```python
from build123d import *

# Parameters (mm, degrees)
SKETCH4_R                = 150
BOSS_EXTRUDE1_DEPTH      = 25
BOSS_EXTRUDE1_DEPTH_BACK = 25
SKETCH4_4_R              = 230
SKETCH4_4_R_2            = 150
BOSS_EXTRUDE2_DEPTH      = 25


with BuildPart() as part:
    # Sketch4 → Boss-Extrude1 (new body, two sides)
    with BuildSketch(Plane.XY) as boss_extrude1_sk:
        with BuildLine():
            Line((71.8245835, 175.909198012), (-101.8245835, 175.909198012))
            ThreePointArc((-101.8245835, 175.909198012), (-480, 0), (-101.8245835, -175.909198012))
            Line((-101.8245835, -175.909198012), (71.8245835, -175.909198012))
            ThreePointArc((71.8245835, -175.909198012), (450, 0), (71.8245835, 175.909198012))
        make_face()
        with Locations((-250, 0)):
            Circle(SKETCH4_R, mode=Mode.SUBTRACT)
        with Locations((220, 0)):
            Circle(SKETCH4_R, mode=Mode.SUBTRACT)
    extrude(amount=BOSS_EXTRUDE1_DEPTH)
    extrude(boss_extrude1_sk.sketch, amount=-BOSS_EXTRUDE1_DEPTH_BACK)

    # Sketch4_4 → Boss-Extrude2 (add)
    with BuildSketch(Plane.XY):
        with Locations((-250, 0)):
            Circle(SKETCH4_4_R)
        with Locations((-250, 0)):
            Circle(SKETCH4_4_R_2, mode=Mode.SUBTRACT)
        with Locations((220, 0)):
            Circle(SKETCH4_4_R)
        with Locations((220, 0)):
            Circle(SKETCH4_4_R_2, mode=Mode.SUBTRACT)
    extrude(amount=-BOSS_EXTRUDE2_DEPTH)


solid = part.part
```
Geometry: final body of the model. Coordinates: model frame, mm. A direction names the side the tool comes from. Coordinates: 2 decimals unless noted, no trailing zeros. Write each loop counter-clockwise with the first axis right and the second up, starting at its lowest first coordinate (ties: lowest second). Pieces come first, ordered by that corner, then holes. Notation, with made-up numbers: M 6.25,82 L 27.25,82 A16 cw 27.25,109 Z; hole C 6.25,36.5 d3. An arc over 180 degrees is marked long. Answer as CSV lines item,"result". Start each with the question number.
Q1. Cut plane B-B on y = -71. Return the cut outline in (x, z), then the cut area to 3 significant figures.
Q2. Reachability of faces 4 (the flat face through (-16, -175.909, 0)), 5 (the flat face through (-14, 175.909, 0)), 6 (the cylindrical face through (-106.93, 45.06, -0.35)) from +Z, -Z, +X, -X, +Y, -Y: full face, straight path, thin tool, end or side. Return the list, or none.
Q3. Mould query, pull axis Y, two halves, no side actions, for faces 1 (the flat face through (-22, 3, 25)), 2 (the cylindrical face through (-479.884, 7.311, 0.35)), 3 (the cylindrical face through (363.07, 45.06, -0.35)). Classes: released by +Y, released by -Y, zero draft, split by the parting line, or undercut.
Q4. Cut plane C-C on z = 16. Return the cut outline in (x, y), then the cut area to 3 significant figures.
Q5. Line query: line 1 (X direction, y = -1, z = 18.5); line 2 (Y direction, x = 220, z = 13.5); line 3 (X direction, y = -12.5, z = 1.5). Output: solid intervals per line, ascending. Write a range as from..to.
Q6. Cut plane A-A on x = 220. Return the cut outline in (y, z), then the cut area to 3 significant figures.
Q7. Cut plane D-D on y = 191.5. Return the cut outline in (x, z).
Q8. Pin query (flat end, axial travel): P1, Ø15, axis at x = 28.5, z = -6, coming from the -Y side; P2, Ø1.5, axis at x = 116, z = 9.5, coming from the -Y side; P3, Ø10, axis at y = -161, z = -12, coming from the +X side. Return the tip coordinate at first contact, or that it passes through.
Findings below:
1,outline,"M -468.77,-25 L -382.13,-25 L -382.13,25 L -468.77,25 Z; M -117.87,-25 L 87.87,-25 L 87.87,25 L -117.87,25 Z; M 352.13,-25 L 438.77,-25 L 438.77,25 L 352.13,25 Z"
1,area,"19,000 mm2"
2,face 4,"+Z, -Z, -Y"
2,face 5,"+Z, -Z, +Y"
2,face 6,"+Z, -Z"
3,face 1,"zero draft"
3,face 2,"split by the parting line"
3,face 3,"undercut"
4,outline,"M -101.82,-175.91 L 71.82,-175.91 A230 ccw long 71.82,175.91 L -101.82,175.91 A230 ccw long Z; hole C -250,0 d300; hole C 220,0 d300"
4,area,"212,000 mm2"
5,line 1,"x = -480..-400, -100..70, 370..450"
5,line 2,"y = -230..-150, 150..230"
5,line 3,"x = -479.66..-399.48, -100.52..70.52, 369.48..449.66"
6,outline,"M -230,-25 L -150,-25 L -150,25 L -230,25 Z; M 150,-25 L 230,-25 L 230,25 L 150,25 Z"
6,area,"8,000 mm2"
7,outline,"M -377.39,-25 L -122.61,-25 L -122.61,25 L -377.39,25 Z; M 92.61,-25 L 347.39,-25 L 347.39,25 L 92.61,25 Z"
8,P1,"stops at y = -175.91"
8,P2,"stops at y = -205.52"
8,P3,"stops at x = 389.01"
